Geometry: final body of the model. Coordinates: model frame, mm. A direction names the side the tool comes from. Coordinates: 2 decimals unless noted, no trailing zeros. Answer as a JSON object with one key per item and string values. Group by question number.
Item 1: Set-up query: faces 1 (the flat face through (-109, -2.5, 105)), 2 (the cylindrical face through (-162.38, -1.23, 132.48)). Return all of +Z, -Z, +X, -X, +Y, -Y with unobstructed straight access to the full face (end or side cutting, diameter ignored); none if empty.
Item 2: Mould query, pull axis Z, two halves, no side actions, for faces 3 (the flat face through (-109, 0, 105)), 4 (the flat face through (234, -1, 164.827)), 5 (the cylindrical face through (-222.79, -1.23, 56.55)). Classes: pulls with the +Z half, pulls with the -Z half, needs draft (parallel to the pull), parting line crosses it, or undercut.
Item 3: Line query: line 1 along Z through (x, y) = (-223.5, -1.5); line 2 along Y through (x, z) = (-230.5, 68); line 3 along X through (y, z) = (-1, 98). Output: solid intervals per line, ascending. Write a range as from..to.
Item 4: First-contact query: pin 1 Ø0.5 at (y, z) = (-1.5, 155) entering from +X; pin 2 Ø2 at (x, y) = (40, -0.5) entering from +Z; pin 3 Ø5 at (x, y) = (3.5, -4) entering from -Z. Flat tips, straight axial feed; report the tip coordinate or a pass-through.
Item 5: Section A-A on z = 121. State how many separate pieces and enclosed holes the cut face has, and give its area (3 significant figures).
```python
from build123d import *

# Parameters (mm, degrees)
F1_DEPTH     = 2.5
F3_D         = 70
F4_D         = 35
F5_W         = 5
F5_H         = 2.5
F6_DEPTH     = 2
F7_DEPTH     = 0.1
F8_T1_DEPTH  = 2.5
F8_T3_DEPTH  = 5
F8_T9_DEPTH  = 21.0404962177
F8_T14_DEPTH = 21.9443021397
F8_T22_DEPTH = 21.0404962177
F8_T27_DEPTH = 21.9443021397


# Not quite as in the source:
# - a fillet or chamfer that OpenCascade refuses, or shapes differently, is made with other operations: its cross-section is extruded or revolved along the edge and cut away or added


with BuildPart() as f1:
    # F0 (on Front) → F1 (new body)
    with BuildSketch(Plane.XZ):
        with BuildLine():
            Line((234.3109268695, 164.7265180945), (-265.6890731305, 164.7265180945))
            Line((-265.6890731305, 164.7265180945), (-265.6890731305, -85.2734819055))
            Line((-265.6890731305, -85.2734819055), (-263.6890731305, -85.2734819055))
            add(Edge.make_bspline(
                [(234.3109268695, 154.7265180945), (-263.6890731305, 154.7265180945), (-263.6890731305, -85.2734819055)],
                knots=[4.7123889804, 4.7123889804, 4.7123889804, 6.2831853072, 6.2831853072, 6.2831853072], degree=2, weights=[1, 0.7071067812, 1]))
            Line((234.3109268695, 154.7265180945), (234.3109268695, 164.7265180945))
        make_face()
    extrude(amount=F1_DEPTH)

    # F3 (through all)
    with Locations(Plane.XZ.offset(2.5)):
        with Locations((-210.6890731305, 109.7265180945)):
            Hole(F3_D / 2)

    # F4 (through all)
    with Locations(Plane.XZ.offset(2.5)):
        with Locations((-145.6890731305, 127.2265180945), (-235.6890731305, 44.7265180945)):
            Hole(F4_D / 2)

    # F5 (on face) → F6 (join)
    with BuildSketch(Plane.XY.offset(164.7265180945)):
        Polygon((239.3109268695, -6.25), (239.3109268695, 3.75), (229.3109268695, 3.75), (229.3109268695, 0), (234.3109268695, 0), (234.3109268695, -2.5), (229.3109268695, -2.5), (229.3109268695, -6.25), align=None)
        with Locations((231.8109268695, -1.25)):
            Rectangle(F5_W, F5_H)
    extrude(amount=-F6_DEPTH)

    # F5 (on face) → F7 (join)
    with BuildSketch(Plane.XY.offset(164.7265180945)):
        Polygon((239.3109268695, -6.25), (239.3109268695, 3.75), (229.3109268695, 3.75), (229.3109268695, 0), (234.3109268695, 0), (234.3109268695, -2.5), (229.3109268695, -2.5), (229.3109268695, -6.25), align=None)
        with Locations((231.8109268695, -1.25)):
            Rectangle(F5_W, F5_H)
    extrude(amount=F7_DEPTH)

    # F8: fillet of radius 8 on 3 edges, made by hand

    # F8_s2 → F8_t1 (join)
    with BuildSketch(Plane.XZ):
        with BuildLine():
            ThreePointArc((234.3109268695, 155.3103196074), (235.6776772888, 159.7824555624), (239.3109268695, 162.7265180945))
            Line((239.3109268695, 162.7265180945), (234.3109268695, 162.7265180945))
            Line((234.3109268695, 162.7265180945), (234.3109268695, 155.3103196074))
        make_face()
    extrude(amount=F8_T1_DEPTH)

    # F8_s4 → F8_t3 (join)
    with BuildSketch(Plane.YZ.offset(229.3109268695)):
        with BuildLine():
            ThreePointArc((-2.5, 155.9487972387), (-3.5, 159.8217805849), (-6.25, 162.7265180945))
            Line((-6.25, 162.7265180945), (-2.5, 162.7265180945))
            Line((-2.5, 162.7265180945), (-2.5, 155.9487972387))
        make_face()
        with BuildLine():
            ThreePointArc((3.75, 162.7265180945), (1, 159.8217805849), (0, 155.9487972387))
            Line((0, 155.9487972387), (0, 162.7265180945))
            Line((0, 162.7265180945), (3.75, 162.7265180945))
        make_face()
    extrude(amount=F8_T3_DEPTH)


with BuildPart() as f8_tool7:
    # F8_s8 → F8_t9 (new body)
    with BuildSketch(Plane.XZ.offset(21.0404962177)):
        with BuildLine():
            ThreePointArc((234.3109268695, 155.3103196074), (235.6776772888, 159.7824555624), (239.3109268695, 162.7265180945))
            Line((239.3109268695, 162.7265180945), (234.3109268695, 162.7265180945))
            Line((234.3109268695, 162.7265180945), (234.3109268695, 155.3103196074))
        make_face()
    extrude(amount=-F8_T9_DEPTH)

    split(bisect_by=Plane.XZ.offset(6.25), keep=Keep.BOTTOM)

    split(bisect_by=Plane.XZ.offset(2.5), keep=Keep.TOP)


with BuildPart() as f8_tool12:
    # F8_s13 → F8_t14 (new body)
    with BuildSketch(Plane.YZ.offset(251.2552290092)):
        with BuildLine():
            ThreePointArc((-2.5, 155.9487972387), (-3.5, 159.8217805849), (-6.25, 162.7265180945))
            Line((-6.25, 162.7265180945), (-2.5, 162.7265180945))
            Line((-2.5, 162.7265180945), (-2.5, 155.9487972387))
        make_face()
    extrude(amount=-F8_T14_DEPTH)

    split(bisect_by=Plane.YZ.offset(234.3109268695), keep=Keep.TOP)

    split(bisect_by=Plane.YZ.offset(239.3109268695), keep=Keep.BOTTOM)


with BuildPart() as f8_tool7_1:
    add(f8_tool7.part)

    # F8_t17: intersect F8_tool12
    add(f8_tool12.part, mode=Mode.INTERSECT)


with BuildPart() as f1_1:
    add(f1.part)

    # F8_t5: union F8_tool7
    add(f8_tool7_1.part)


with BuildPart() as f8_tool20:
    # F8_s21 → F8_t22 (new body)
    with BuildSketch(Plane.XZ.offset(2.5)):
        with BuildLine():
            ThreePointArc((234.3109268695, 155.3103196074), (235.6776772888, 159.7824555624), (239.3109268695, 162.7265180945))
            Line((239.3109268695, 162.7265180945), (234.3109268695, 162.7265180945))
            Line((234.3109268695, 162.7265180945), (234.3109268695, 155.3103196074))
        make_face()
    extrude(amount=-F8_T22_DEPTH)

    split(bisect_by=Plane.XZ.offset(-3.75), keep=Keep.TOP)

    split(bisect_by=Plane.XZ, keep=Keep.BOTTOM)


with BuildPart() as f8_tool25:
    # F8_s26 → F8_t27 (new body)
    with BuildSketch(Plane.YZ.offset(251.2552290092)):
        with BuildLine():
            ThreePointArc((3.75, 162.7265180945), (1, 159.8217805849), (0, 155.9487972387))
            Line((0, 155.9487972387), (0, 162.7265180945))
            Line((0, 162.7265180945), (3.75, 162.7265180945))
        make_face()
    extrude(amount=-F8_T27_DEPTH)

    split(bisect_by=Plane.YZ.offset(234.3109268695), keep=Keep.TOP)

    split(bisect_by=Plane.YZ.offset(239.3109268695), keep=Keep.BOTTOM)


with BuildPart() as f8_tool20_1:
    add(f8_tool20.part)

    # F8_t30: intersect F8_tool25
    add(f8_tool25.part, mode=Mode.INTERSECT)


with BuildPart() as f1_2:
    add(f1_1.part)

    # F8_t18: union F8_tool20
    add(f8_tool20_1.part)


solid = f1_2.part
```
Checks:
{
 "1": {"face 1": "+Z, -Z, -X, -Y", "face 2": "+Y, -Y"},
 "2": {"face 3": "needs draft", "face 4": "pulls with the +Z half", "face 5": "undercut"},
 "3": {"line 1": "9.18..32.17, 57.28..77.16, 142.3..164.73", "line 2": "-2.5..0", "line 3": "-265.69..-243.67, -177.71..-87.22"},
 "4": {"pin 1": "x = 234.31", "pin 2": "z = 164.73", "pin 3": "z = 126.89"},
 "5": {"separate pieces": "3", "enclosed holes": "0", "area": "366 mm^2"}
}
